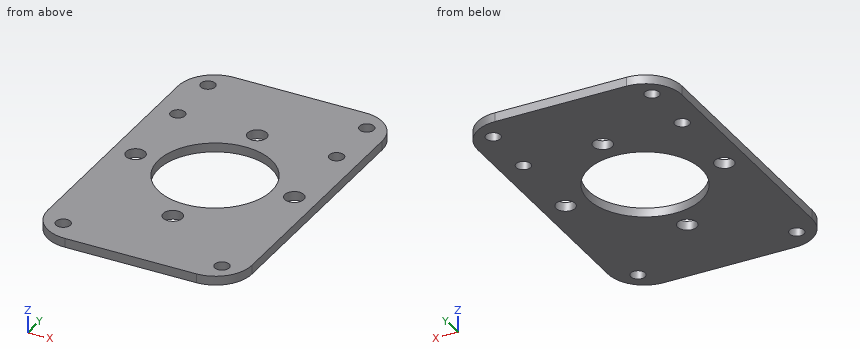
from build123d import *

# Parameters (mm, degrees)
SKETCH_1_W      = 45
SKETCH_1_H      = 70
SKETCH_1_R      = 2.1
SKETCH_1_R_2    = 12.5
SKETCH_1_R_3    = 1.6
EXTRUDE_1_DEPTH = 2
FILLET_1_R      = 8


with BuildPart() as part:
    # ｽｹｯﾁ1 → ﾎﾞｽ - 押し出し1 (new body)
    with BuildSketch(Plane.XY):
        Rectangle(SKETCH_1_W, SKETCH_1_H)
        with Locations((-17.5, 0)):
            Circle(SKETCH_1_R, mode=Mode.SUBTRACT)
        with Locations((0, 17.5)):
            Circle(SKETCH_1_R, mode=Mode.SUBTRACT)
        with Locations((17.5, 0)):
            Circle(SKETCH_1_R, mode=Mode.SUBTRACT)
        with Locations((0, -17.5)):
            Circle(SKETCH_1_R, mode=Mode.SUBTRACT)
        Circle(SKETCH_1_R_2, mode=Mode.SUBTRACT)
        with Locations((-17.5, 30)):
            Circle(SKETCH_1_R_3, mode=Mode.SUBTRACT)
        with Locations((17.5, 30)):
            Circle(SKETCH_1_R_3, mode=Mode.SUBTRACT)
        with Locations((-17.5, -30)):
            Circle(SKETCH_1_R_3, mode=Mode.SUBTRACT)
        with Locations((17.5, -30)):
            Circle(SKETCH_1_R_3, mode=Mode.SUBTRACT)
        with Locations((-17.5, 17.5)):
            Circle(SKETCH_1_R_3, mode=Mode.SUBTRACT)
        with Locations((17.5, 17.5)):
            Circle(SKETCH_1_R_3, mode=Mode.SUBTRACT)
    extrude(amount=EXTRUDE_1_DEPTH)

    # ﾌｨﾚｯﾄ1
    fillet_1_edges = [part.edges().sort_by_distance(p)[0] for p in [
        (-22.5, 35, 1),
        (22.5, 35, 1),
        (22.5, -35, 1),
        (-22.5, -35, 1),
    ]]
    fillet(fillet_1_edges, radius=FILLET_1_R)


solid = part.part
Geometry check sheet. Reference: the model listing, model coordinates, mm. Coordinates: 2 decimals unless noted, no trailing zeros. Order: outer loops, then holes, each group sorted by start corner. A loop starts at its lowest first (then second) coordinate and runs counter-clockwise, first axis right, second up. Notation, with made-up numbers: (38.25, 40) - (50.25, 40) arc R23 ccw to (50.25, 59) - close; hole circle Ø11 at (84, -15). An arc over 180 degrees is marked (long way). Answer in a Markdown table with one row per item. Add a question column.
1) Cross-section at C-C, the plane z = 0.9. State how many separate pieces and enclosed holes the cut face has, then the cut area to 3 significant figures.
2) Cross-section at B-B, the plane y = 17.5. Record the cut outline in (x, z), then the cut area to 3 significant figures.
3) Cross-section at D-D, the plane x = -17.5. Record the cut outline in (y, z), then the cut area to 3 significant figures.
4) Gauge pin test, flat end, axial feed: P1, Ø3.5, axis at x = 17.5, y = 0, coming from the -Z side. Record the tip position at first contact, or that the pin passes through.
5) Material ranges on line 1 along Y through (x, z) = (0, 1.4); line 2 along Y through (x, z) = (-17.5, 1.1); line 3 along Y through (x, z) = (-17, 0.2), recorded low to high. Write a range as [from, to].
6) Cross-section at A-A, the plane x = 0. Record the cut outline in (y, z), then the cut area to 3 significant figures.
Check result:
| question | item | result |
|---|---|---|
| 1 | separate pieces | 1 |
| 1 | enclosed holes | 11 |
| 1 | area | 2,500 mm² |
| 2 | outline | (-22.5, 0) - (-19.1, 0) - (-19.1, 2) - (-22.5, 2) - close; (-15.9, 0) - (-2.1, 0) - (-2.1, 2) - (-15.9, 2) - close; (2.1, 0) - (15.9, 0) - (15.9, 2) - (2.1, 2) - close; (19.1, 0) - (22.5, 0) - (22.5, 2) - (19.1, 2) - close |
| 2 | area | 68.8 mm² |
| 3 | outline | (-34.42, 0) - (-31.6, 0) - (-31.6, 2) - (-34.42, 2) - close; (-28.4, 0) - (-2.1, 0) - (-2.1, 2) - (-28.4, 2) - close; (2.1, 0) - (15.9, 0) - (15.9, 2) - (2.1, 2) - close; (19.1, 0) - (28.4, 0) - (28.4, 2) - (19.1, 2) - close; (31.6, 0) - (34.42, 0) - (34.42, 2) - (31.6, 2) - close |
| 3 | area | 110 mm² |
| 4 | P1 | passes through |
| 5 | line 1 | y = [-35, -19.6], [-15.4, -12.5], [12.5, 15.4], [19.6, 35] |
| 5 | line 2 | y = [-34.42, -31.6], [-28.4, -2.1], [2.1, 15.9], [19.1, 28.4], [31.6, 34.42] |
| 5 | line 3 | y = [-34.6, -31.52], [-28.48, -2.04], [2.04, 15.98], [19.02, 28.48], [31.52, 34.6] |
| 6 | outline | (-35, 0) - (-19.6, 0) - (-19.6, 2) - (-35, 2) - close; (-15.4, 0) - (-12.5, 0) - (-12.5, 2) - (-15.4, 2) - close; (12.5, 0) - (15.4, 0) - (15.4, 2) - (12.5, 2) - close; (19.6, 0) - (35, 0) - (35, 2) - (19.6, 2) - close |
| 6 | area | 73.2 mm² |
